from build123d import *

# Parameters (mm, degrees)
ESQUISSE1_W             = 186
ESQUISSE1_H             = 132
BOSS_EXTRU_1_DEPTH      = 3
ESQUISSE4_W             = 5
ESQUISSE4_H             = 122
BOSS_EXTRU_4_DEPTH      = 50
ESQUISSE5_W             = 126
ESQUISSE5_H             = 7
ENL_V_MAT_EXTRU_1_DEPTH = 183


with BuildPart() as part:
    # Esquisse1 → Boss.-Extru.1 (new body)
    with BuildSketch(Plane(origin=(0, 0, 0), x_dir=(1, 0, 0), z_dir=(0, 1, 0))):
        Rectangle(ESQUISSE1_W, ESQUISSE1_H)
    extrude(amount=BOSS_EXTRU_1_DEPTH)

    # Esquisse4 → Boss.-Extru.4 (add)
    with BuildSketch(Plane(origin=(0, 3, 0), x_dir=(1, 0, 0), z_dir=(0, 1, 0))):
        Polygon((93, 61), (93, 66), (-93, 66), (-93, 61), (-88, 61), align=None)
        with Locations((-90.5, 0)):
            Rectangle(ESQUISSE4_W, ESQUISSE4_H)
        Polygon((93, -66), (93, -61), (-88, -61), (-93, -61), (-93, -66), align=None)
    extrude(amount=BOSS_EXTRU_4_DEPTH)

    # Esquisse5 → Enlèv. mat.-Extru.1 (cut)
    with BuildSketch(Plane(origin=(93, 0, 0), x_dir=(0, 0, -1), z_dir=(1, 0, 0))):
        with Locations((0, 46.5)):
            Rectangle(ESQUISSE5_W, ESQUISSE5_H)
    extrude(amount=-ENL_V_MAT_EXTRU_1_DEPTH, mode=Mode.SUBTRACT)


solid = part.part
Can you work these out from the model? Positions are in its coordinate system, mm. A direction names the side the tool comes from. Coordinates: 2 decimals unless noted, no trailing zeros. Write each loop counter-clockwise with the first axis right and the second up, starting at its lowest first coordinate (ties: lowest second). Pieces come first, ordered by that corner, then holes. Notation, with made-up numbers: (60.25, 8) -> (65.25, 8) arc R16 cw to (65.25, 39) -> close; hole circle Ø2 at (6, -37.75). An arc over 180 degrees is marked (long way). Write each question's results on one line, items separated by ' | '. Start each with the question number.
Q1. Imagine slicing it at B-B (y = 48). Write out the boundary of the cut face in (x, z).
Q2. I'm going to push flat-ended pins straight in: pin 1 (20 mm diameter, centred on y = 26, z = -27, fed in from +X); pin 2 (5.5 mm diameter, centred on y = 46.5, z = 1.5, fed in from +X). Where does each tip first touch, or does it pass through?
Q3. Imagine slicing it at C-C (z = -5). Write out the boundary of the cut face in (x, y), then the cut area to 3 significant figures.
Q4. On a 3-axis mill with a long thin cutter (end or side, diameter ignored), from which of +Z, -Z, +X, -X, +Y, -Y can I reach the whole of each face in a straight line? I mean faces 4 (the face through (3, 46, 63)), 5 (the face through (93, 2.8, 5.2)), 6 (the face through (1, 23, -61)). Say none if no direction works.
Q5. Imagine slicing it at A-A (x = 6). Write out the boundary of the cut face in (y, z), then the cut area to 3 significant figures.
Q6. We'd pull the mould along Z, two halves only. Please class faces 1 (the face through (-88, 23, 1)), 2 (the face through (-1, 0, -1)), 3 (the face through (1, 26, -66)): +Z half, -Z half, draft (parallel to the pull), parting line (faces both ways), or undercut.
Q7. If I drill on probe 1 along Z at (x, y) = (77, 29); probe 2 along Z at (x, y) = (52.5, 47); probe 3 along Y at (x, z) = (-65.5, 16), over which ranges is the centre line in solid material (lowest first)?
Q8. Imagine slicing it at D-D (y = 16). Write out the boundary of the cut face in (x, z).
Taken from the geometry:
1) outline: (-93, -66) -> (93, -66) -> (93, -63) -> (-90, -63) -> (-90, 63) -> (93, 63) -> (93, 66) -> (-93, 66) -> close
2) pin 1: stops at x = -88 | pin 2: stops at x = -90
3) outline: (-93, 0) -> (93, 0) -> (93, 3) -> (-88, 3) -> (-88, 43) -> (-90, 43) -> (-90, 50) -> (-88, 50) -> (-88, 53) -> (-93, 53) -> close | area: 794 mm^2
4) face 4: +X | face 5: +Z, -Z, +X, +Y, -Y | face 6: +X, +Y
5) outline: (0, -66) -> (53, -66) -> (53, -61) -> (50, -61) -> (50, -63) -> (43, -63) -> (43, -61) -> (3, -61) -> (3, 61) -> (43, 61) -> (43, 63) -> (50, 63) -> (50, 61) -> (53, 61) -> (53, 66) -> (0, 66) -> close | area: 868 mm^2
6) face 1: undercut | face 2: draft | face 3: -Z half
7) probe 1: z = -66 to -61, 61 to 66 | probe 2: z = -66 to -63, 63 to 66 | probe 3: y = 0 to 3
8) outline: (-93, -66) -> (93, -66) -> (93, -61) -> (-88, -61) -> (-88, 61) -> (93, 61) -> (93, 66) -> (-93, 66) -> close
